from build123d import *

# Parameters (mm, degrees)
F0_R     = 3
F1_DEPTH = 14
F3_DEPTH = 3
F4_R     = 3
F5_DEPTH = 7
F6_R     = 1
F8_R     = 2
F10_SIZE = 1


# Not quite as in the source:
# - an extrude whose draft closes it to a point is written as a loft to that point


with BuildPart() as f1:
    # F0 (on Top) → F1 (new body)
    with BuildSketch(Plane.XY):
        Circle(F0_R)
    extrude(amount=F1_DEPTH)

    # F2 (on face) → F3 (join)
    with BuildSketch(Plane.XY.offset(14)):
        with BuildLine():
            Line((-5, 3.3166247904), (-5, -3.3166247904))
            ThreePointArc((-5, -3.3166247904), (0, -6), (5, -3.3166247904))
            Line((5, -3.3166247904), (5, 3.3166247904))
            ThreePointArc((5, 3.3166247904), (0, 6), (-5, 3.3166247904))
        make_face()
    extrude(amount=F3_DEPTH)

    # F4 (on face) → F5 (join)
    with BuildSketch(Plane.XY.offset(17)):
        Circle(F4_R)
    extrude(amount=F5_DEPTH)

    # F6
    f6_edges = [f1.edges().sort_by_distance(p)[0] for p in [
        (-3, 0, 24),
    ]]
    fillet(f6_edges, radius=F6_R)

    # F8 (on offset) → F9 section 0
    with BuildSketch(Plane.YZ.offset(3), mode=Mode.PRIVATE) as f9_s0:
        with Locations((0, 7.2)):
            Circle(F8_R)
    loft([f9_s0.sketch, Vertex(1, 0, 7.2)], ruled=True, mode=Mode.SUBTRACT)

    # F10
    f10_edges = [f1.edges().sort_by_distance(p)[0] for p in [
        (-3, 0, 0),
    ]]
    chamfer(f10_edges, length=F10_SIZE)


solid = f1.part
Check sheet for the modelled part. Datum: model origin and axes. Units: mm. A direction names the side the tool comes from. Round coordinates to 2 decimals unless told otherwise and drop trailing zeros. Order: outer loops, then holes, each group sorted by start corner. A loop starts at its lowest first (then second) coordinate and runs counter-clockwise, first axis right, second up.
(1) Draft check along Z on faces 1 (the conical face through (1.5, -0.5, 7.2)), 2 (the cylindrical face through (-3, 0, 7)), 3 (the flat face through (3.3, 0.1, 17)). Enter one of: pulls with the +Z half, pulls with the -Z half, needs draft (parallel to the pull), parting line crosses it, or undercut.
(2) Go/stop test with flat-tipped pins: P1, Ø1.5, axis at x = -3, z = 20.5, coming from the +Y side; P2, Ø1.5, axis at x = 3, y = 2.5, coming from the +Z side; P3, Ø1, axis at x = 3, z = 12, coming from the -Y side. Record where each tip stops, or that it passes through.
(3) Cross-section at A-A, the plane x = 0. Enter the section's corners in (y, z), and give its area (3 significant figures).
(4) Access from +Z, -Z, +X, -X, +Y, -Y to the whole of each face (thin tool, end or side, straight path). Record for faces 4 (the flat face through (0, 0, 24)), 5 (the flat face through (3.3, 0.1, 14)), 6 (the cylindrical face through (-3, 0, 20)).
(5) Cross-section at C-C, the plane x = 3.25. Enter the section's corners in (y, z), and give its area (3 significant figures).
(6) Scan lines: probe 1 along Z at (x, y) = (-4.25, 3.75); probe 2 along Y at (x, z) = (2.25, 19.5); probe 3 along X at (y, z) = (5, 15.75). Record each from-to range of solid material in increasing order.
(7) Cross-section at B-B, the plane z = 1.5. Enter the section's corners in (x, y), and give its area (3 significant figures).
Check sheet entries:
1. face 1: undercut
1. face 2: needs draft
1. face 3: pulls with the +Z half
2. P1: stops at y = 1.98
2. P2: stops at z = 17
2. P3: stops at y = -1.66
3. outline: (-6, 14) - (-3, 14) - (-3, 1) - (-2, 0) - (2, 0) - (3, 1) - (3, 14) - (6, 14) - (6, 17) - (3, 17) - (3, 23) arc R1 ccw to (2, 24) - (-2, 24) arc R1 ccw to (-3, 23) - (-3, 17) - (-6, 17) - close
3. area: 161 mm2
4. face 4: +Z, +X, -X, +Y, -Y
4. face 5: -Z
4. face 6: +Z
5. outline: (-5.04, 14) - (5.04, 14) - (5.04, 17) - (-5.04, 17) - close
5. area: 30.3 mm2
6. probe 1: z = 14 to 17
6. probe 2: y = -1.98 to 1.98
6. probe 3: x = -3.32 to 3.32
7. outline: circle Ø6 at (0, 0)
7. area: 28.3 mm2
